The drawing under review shows one solid part. Ordinate dimensions are in mm from its lowest x, y, z. Coordinates: 2 decimals unless noted, no trailing zeros. Write each loop counter-clockwise with the first axis right and the second up, starting at its lowest first coordinate (ties: lowest second). Pieces come first, ordered by that corner, then holes.
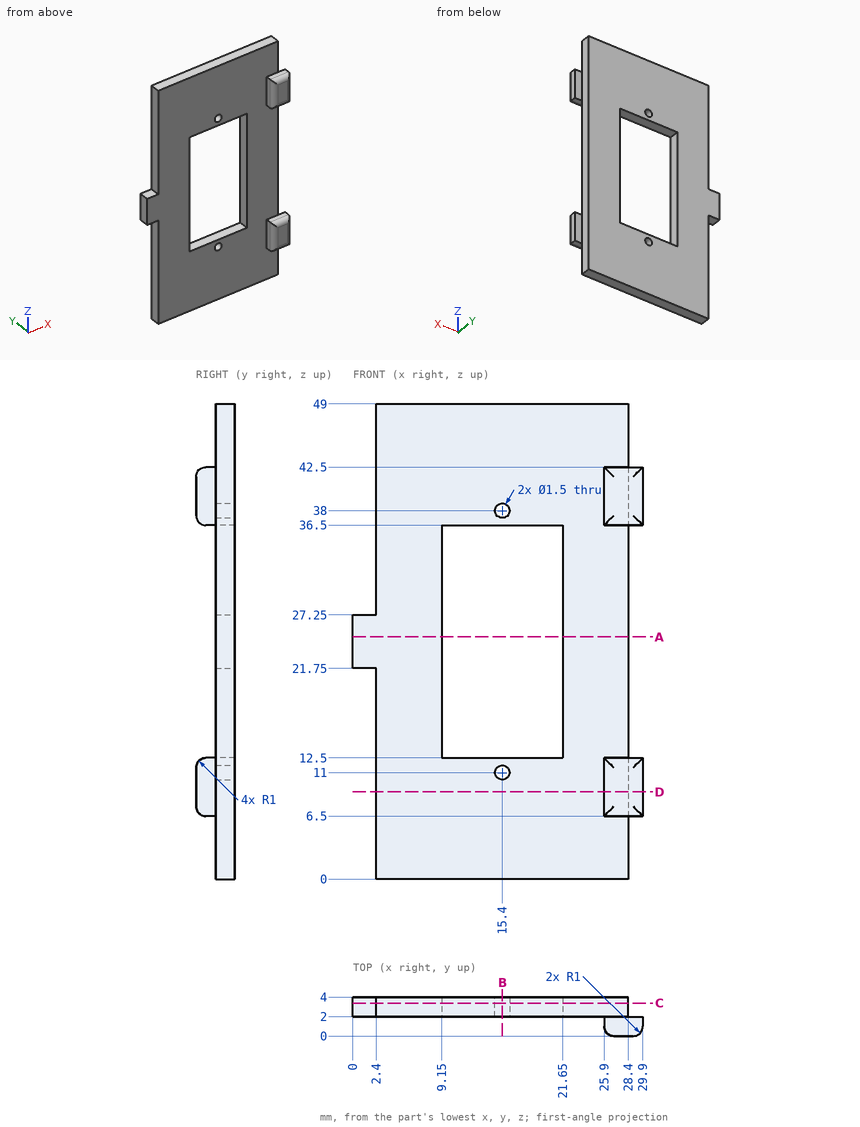
Q1. Add section C-C (y = 3.4). State the section outline as (x, z) points, then the cut area to 3 significant figures.
Ans:
outline: (0, 21.75) - (2.4, 21.75) - (2.4, 0) - (28.4, 0) - (28.4, 49) - (2.4, 49) - (2.4, 27.25) - (0, 27.25) - close; hole (9.15, 12.5) - (21.65, 12.5) - (21.65, 36.5) - (9.15, 36.5) - close; hole circle Ø1.5 at (15.4, 11); hole circle Ø1.5 at (15.4, 38)
area: 984 mm2
Q2. Add section A-A (z = 25). State the section outline as (x, y) points, then the cut area to 3 significant figures.
Ans:
outline: (0, 2) - (9.15, 2) - (9.15, 4) - (0, 4) - close; (21.65, 2) - (28.4, 2) - (28.4, 4) - (21.65, 4) - close
area: 31.8 mm2
Q3. For probe 1 along Z at (x, y) = (15.4, 3.3); probe 2 along X at (y, z) = (2.5, 11); probe 3 along Z at (x, y) = (12.25, 3.2), list the stretches that pass through material, from the lowest coordinate up.
Ans:
probe 1: z = 0 to 10.25, 11.75 to 12.5, 36.5 to 37.25, 38.75 to 49
probe 2: x = 2.4 to 14.65, 16.15 to 28.4
probe 3: z = 0 to 12.5, 36.5 to 49
Q4. Add section B-B (x = 15.4). State the section outline as (y, z) points, then the cut area to 3 significant figures.
Ans:
outline: (2, 0) - (4, 0) - (4, 10.25) - (2, 10.25) - close; (2, 11.75) - (4, 11.75) - (4, 12.5) - (2, 12.5) - close; (2, 36.5) - (4, 36.5) - (4, 37.25) - (2, 37.25) - close; (2, 38.75) - (4, 38.75) - (4, 49) - (2, 49) - close
area: 44.0 mm2
Q5. Add section D-D (z = 9). State the section outline as (x, y) points.
Ans:
outline: (2.4, 2) - (25.9, 2) - (25.9, 1) arc R1 ccw to (26.9, 0) - (28.9, 0) arc R1 ccw to (29.9, 1) - (29.9, 2) - (28.4, 2) - (28.4, 4) - (2.4, 4) - close
Q6. Clearance check with flat-ended pins moving along their axes: pin 1 Ø0.8 at (x, y) = (28, 1.5) entering from +Z; pin 2 Ø0.5 at (x, y) = (28, 1.5) entering from -Z; pin 3 Ø1.6 at (y, z) = (3, 30.5) entering from +X. State where each tip first meets the part, or that it passes through.
Ans:
pin 1: stops at z = 42.5
pin 2: stops at z = 6.5
pin 3: stops at x = 28.4
